Read the model definition and answer for the solid it produces. Units are mm, in the model's axes. A direction names the side the tool comes from. Coordinates: 2 decimals unless noted, no trailing zeros. Loops run counter-clockwise (first coordinate to the right, second up) from the corner with the lowest first, then second, coordinate; pieces in that order, holes last. Notation, with made-up numbers: M 13,27 L 21,27 A13 ccw 21,51 Z; hole C 49,-23 d9. An arc over 180 degrees is marked long. Use one line per item in the form item = value. Start each with the question number.
1. The part is cut by section B-B (x = 17.25). Give the vertices of the cut face in (y, z).
2. Flat-ended cylindrical pins translate along their axes: pin 1 (4 mm diameter, centred on x = 13, y = -30.5, fed in from +Z); pin 2 (4 mm diameter, centred on x = 7, z = -96, fed in from -Y); pin 3 (1.5 mm diameter, centred on x = -0.5, y = -23.5, fed in from -Z). Find the tip coordinate at first contact, or state that the pin passes through.
3. A tool of negligible diameter and unlimited length cuts with its end or side. For faces 1 (the flat face through (16, -11, -52)), 2 (the flat face through (8, -41.1, -87)), 3 (the flat face through (8, -37.7, -39)), 4 (the cylindrical face through (8.1, -42.9, -93.2)), 5 (the flat face through (0, -11, -52)), from which of +Z, -Z, +X, -X, +Y, -Y can it reach the whole face along a straight path? Write none if from no direction.
4. The part is cut by section C-C (y = -21.5). Give the vertices of the cut face in (x, z).
5. For a pull along Y with two mould halves and no side action, classify faces 6 (the flat face through (8, -17, -56.5)), 7 (the flat face through (8, 10, -51)), 8 (the flat face through (3.7, -43, -102)) as released by +Y, released by -Y, zero draft, split by the parting line, or undercut.
6. The part is cut by section D-D (x = 5.75). Give the vertices of the cut face in (y, z).
7. Find the intervals of material crossed by probe 1 along Y at (x, z) = (10, -23); probe 2 along Y at (x, z) = (1.75, -46); probe 3 along X at (y, z) = (5.5, -58), in increasing order. Write a range as [from, to].
8. The part is cut by section A-A (z = -32). Give the vertices of the cut face in (x, y).
from build123d import *

# Parameters (mm, degrees)
EXTRUDE_1_DEPTH     = 16
CUT_EXTRUDE_1_DEPTH = 3
EXTRUDE_START       = -44.7
EXTRUDE_2_DEPTH     = 7
CUT_EXTRUDE_START   = -44.7
CUT_EXTRUDE_2_DEPTH = 7
SKETCH_4_W          = 33.124722218
SKETCH_4_H          = 3.4
CUT_EXTRUDE_3_DEPTH = 25
CUT_EXTRUDE_4_REACH = 79.827
SKETCH_6_R          = 0.74


# Read off the part's stored shape, not the designer's step: the extrude step, the extrude step
with BuildPart() as part:
    # Sketch 1 → Extrude 1 (new body)
    with BuildSketch(Plane(origin=(0, 0, 0), x_dir=(0, 0, -1), z_dir=(1, 0, 0))):
        Polygon((0, 0), (13, 0), (13, 3), (47.5, 3), (47.5, -37.7), (0, -37.7), (0, -44.7), (52, -44.7), (52, 10), (0, 10), align=None)
    extrude_1 = extrude(amount=EXTRUDE_1_DEPTH)

    # Sketch 2 → Cut-Extrude 1 (cut)
    with BuildSketch(Plane.XZ):
        with BuildLine():
            Line((8, 0), (0, 0))
            Line((0, 0), (0, -6.5))
            Line((0, -6.5), (0, -13))
            Line((0, -13), (8.000000017, -13))
            ThreePointArc((8.000000017, -13), (1.5, -6.500000009), (8, 0))
        make_face()
        with BuildLine():
            Line((16, 0), (8, 0))
            ThreePointArc((8, 0), (12.596194078, -1.903805922), (14.5, -6.5))
            ThreePointArc((14.5, -6.5), (12.596194084, -11.096194072), (8.000000017, -13))
            Line((8.000000017, -13), (16, -13))
            Line((16, -13), (16, 0))
        make_face()
    cut_extrude_1 = extrude(amount=-CUT_EXTRUDE_1_DEPTH, mode=Mode.SUBTRACT)

    # Extrude 2 outline → Extrude 2 (add)
    with BuildSketch(Plane(origin=(0, 0, 0), x_dir=(1, 0, 0), z_dir=(0, 1, 0)).offset(EXTRUDE_START)):
        with BuildLine():
            ThreePointArc((0, 14.049834435), (8, -4.5), (16, 14.049834435))
            Line((16, 14.049834435), (16, 0))
            Line((16, 0), (0, 0))
            Line((0, 0), (0, 14.049834435))
        make_face()
    extrude_2 = extrude(amount=EXTRUDE_2_DEPTH)

    # Cut-Extrude 2 outline → Cut-Extrude 2 (cut)
    with BuildSketch(Plane(origin=(0, 0, 0), x_dir=(1, 0, 0), z_dir=(0, 1, 0)).offset(CUT_EXTRUDE_START)):
        with BuildLine():
            ThreePointArc((12.3, 6.5), (8, 10.8), (3.7, 6.5))
            Line((3.7, 6.5), (3.7, -3.624722218))
            ThreePointArc((3.7, -3.624722218), (8, -4.5), (12.3, -3.624722218))
            Line((12.3, -3.624722218), (12.3, 6.5))
        make_face()
    cut_extrude_2 = extrude(amount=CUT_EXTRUDE_2_DEPTH, mode=Mode.SUBTRACT)

    # Sketch 4 → Cut-Extrude 3 (cut, symmetric)
    with BuildSketch(Plane.ZY):
        with Locations((-12.937638891, -39.4)):
            Rectangle(SKETCH_4_W, SKETCH_4_H)
    cut_extrude_3 = extrude(amount=CUT_EXTRUDE_3_DEPTH, both=True, mode=Mode.SUBTRACT)

    # Sketch 6 → Cut-Extrude 4 (cut, up to next)
    with BuildSketch(Plane.XZ.offset(44.7), mode=Mode.PRIVATE) as cut_extrude_4_sk1:
        with Locations(Location((0.90598139, -6.208624029, 0), (0, 0, 270))):
            Circle(SKETCH_6_R)
    cut_extrude_4_tool1 = extrude(cut_extrude_4_sk1.sketch, amount=-CUT_EXTRUDE_4_REACH, mode=Mode.PRIVATE) & part.part
    # Sketch 6 → Cut-Extrude 4 (cut, up to next)
    with BuildSketch(Plane.XZ.offset(44.7), mode=Mode.PRIVATE) as cut_extrude_4_sk2:
        with Locations(Location((7.708624029, -13.59401861, 0), (0, 0, 270))):
            Circle(SKETCH_6_R)
    cut_extrude_4_tool2 = extrude(cut_extrude_4_sk2.sketch, amount=-CUT_EXTRUDE_4_REACH, mode=Mode.PRIVATE) & part.part
    # Sketch 6 → Cut-Extrude 4 (cut, up to next)
    with BuildSketch(Plane.XZ.offset(44.7), mode=Mode.PRIVATE) as cut_extrude_4_sk3:
        with Locations(Location((15.09401861, -6.791375971, 0), (0, 0, 270))):
            Circle(SKETCH_6_R)
    cut_extrude_4_tool3 = extrude(cut_extrude_4_sk3.sketch, amount=-CUT_EXTRUDE_4_REACH, mode=Mode.PRIVATE) & part.part
    cut_extrude_4_1 = cut_extrude_4_tool1.solids().sort_by_distance((0.905981, -44.7, -6.208624))[0]
    add(cut_extrude_4_1, mode=Mode.SUBTRACT)
    cut_extrude_4_2 = cut_extrude_4_tool2.solids().sort_by_distance((7.708624, -44.7, -13.594019))[0]
    add(cut_extrude_4_2, mode=Mode.SUBTRACT)
    cut_extrude_4_3 = cut_extrude_4_tool3.solids().sort_by_distance((15.094019, -44.7, -6.791376))[0]
    add(cut_extrude_4_3, mode=Mode.SUBTRACT)
    cut_extrude_4 = cut_extrude_4_1 + cut_extrude_4_2 + cut_extrude_4_3  # Cut-Extrude 4 as one shape, for the pattern or mirror that repeats it

    # Mirror 1: Extrude 1, Cut-Extrude 1, Extrude 2, Cut-Extrude 2, Cut-Extrude 3, Cut-Extrude 4 across plane
    add(extrude_1.mirror(Plane(origin=(16, -44.7, -52), x_dir=(1, 0, 0), z_dir=(0, 0, 1))))
    add(cut_extrude_1.mirror(Plane(origin=(16, -44.7, -52), x_dir=(1, 0, 0), z_dir=(0, 0, 1))), mode=Mode.SUBTRACT)
    add(extrude_2.mirror(Plane(origin=(16, -44.7, -52), x_dir=(1, 0, 0), z_dir=(0, 0, 1))))
    add(cut_extrude_2.mirror(Plane(origin=(16, -44.7, -52), x_dir=(1, 0, 0), z_dir=(0, 0, 1))), mode=Mode.SUBTRACT)
    add(cut_extrude_3.mirror(Plane(origin=(16, -44.7, -52), x_dir=(1, 0, 0), z_dir=(0, 0, 1))), mode=Mode.SUBTRACT)
    add(cut_extrude_4.mirror(Plane(origin=(16, -44.7, -52), x_dir=(1, 0, 0), z_dir=(0, 0, 1))), mode=Mode.SUBTRACT)


solid = part.part
Computed values:
q1.outline = M -44.7,-103.45 L -41.1,-103.45 L -41.1,-91.55 L -44.7,-91.55 Z; M -44.7,-12.45 L -41.1,-12.45 L -41.1,-0.55 L -44.7,-0.55 Z
q2.pin_1 = -47.5
q2.pin_2 = 0
q2.pin_3 = -56.5
q3.face_1 = +X, +Y
q3.face_2 = -Z, +X, -X
q3.face_3 = +Z, +X, -X
q3.face_4 = -Z, -Y
q3.face_5 = -X, +Y
q4.outline = M 0,-56.5 L 16,-56.5 L 16,-47.5 L 0,-47.5 Z
q5.face_6 = undercut
q5.face_7 = released by +Y
q5.face_8 = zero draft
q6.outline = M -44.7,-93.84 L -41.1,-93.84 L -41.1,-74.5 L -37.7,-74.5 L -37.7,-56.5 L 3,-56.5 L 3,-91.4 L 0,-91.4 L 0,-103.6 L 3,-103.6 L 3,-104 L 10,-104 L 10,0 L 3,0 L 3,-0.4 L 0,-0.4 L 0,-12.6 L 3,-12.6 L 3,-47.5 L -37.7,-47.5 L -37.7,-29.5 L -41.1,-29.5 L -41.1,-10.16 L -44.7,-10.16 Z
q7.probe_1 = [-44.7, -41.1], [3, 10]
q7.probe_2 = [-44.7, -37.7], [3, 10]
q7.probe_3 = [0, 16]
q8.outline = M 0,-44.7 L 16,-44.7 L 16,-37.7 L 0,-37.7 Z; M 0,3 L 16,3 L 16,10 L 0,10 Z
